from build123d import *

# Parameters (mm, degrees)
F0_R     = 2.1855866809
F1_DEPTH = 3.048


with BuildPart() as f1:
    # F0 (on Front) → F1 (new body)
    with BuildSketch(Plane.XZ):
        Polygon((-5.9369264533, -6.6248892115), (-8.0986570849, -26.090829358), (-8.0986570849, -29.0724959499), (-6.7978715524, -28.209612886), (-3.9593786933, -29.0724959499), (0, -28.209612886), (0, -5.0586252473), (4.1217724793, -0.9782924317), (1.2832815992, -8.4293344989), (5.1818756491, -2.3217138641), (1.8154965946, -11.4109388133), (5.7322757336, -6.8417807078), (2.702526981, -15.0221036917), (5.7322757336, -11.4109388133), (3.0573392287, -18.6332685701), (6.4980270698, -14.4673358305), (3.4121514764, -22.7992013097), (8.4402870655, -15.2195461217), (11.2180029973, -7.7197118662), (9.9174999541, 0), (5.0088027492, 10.0208651274), (8.024699986, 4.6986923553), (8.024699986, 10.0208651274), (9.9174999541, 2.5698228274), (9.9174999541, 8.0731014378), (12.9247023214, 1.6827941872), (12.9247023214, 7.682890673), (16.5401790291, 0), (16.5401790291, 5.5857207626), (18.9088093805, -2.7523501776), (18.9088093805, 2.0773874768), (21.6825364495, -3.8167845923), (21.6825364495, 0), (24.3970053162, -5.7682483457), (24.3970053162, 0), (21.6849464923, 5.7631270029), (17.9872654723, 10.3869775868), (13.3964173922, 12.7771075341), (7.8472970054, 15.6661421061), (14.1803448269, 14.6780370192), (12.2824395075, 15.6661421061), (20.1555828001, 13.5067671671), (16.00795798, 15.6661421061), (23.2676268034, 14.7984231008), (26.9920900816, 12.8593584523), (24.7008390725, 15.6661421061), (29.2833410908, 13.2803573629), (25.9918076559, 18.5046344995), (19.2012600601, 21.019651712), (14.9435270578, 21.019651712), (9.621351026, 21.019651712), (1.8154965946, 18.5046344995), (7.3503633432, 22.9420375162), (4.2991787195, 21.019651712), (7.6698875055, 25.0856313896), (2.8167848962, 22.9420375162), (9.621351026, 27.229225263), (4.6539907344, 27.229225263), (11.2102990657, 29.3158966176), (9.621351026, 29.9043957943), (12.7992471054, 31.9066156085), (9.621351026, 33.0836139619), (1.3918339066, 27.8986419471), (-2.087427536, 18.5046344995), (-3.3292702865, 24.9229501933), (-7.3300888762, 30.5999331176), (-14.4263189286, 35.2124832571), (-23.553526029, 35.2124832571), (-14.4263189286, 33.4919277449), (-19.5913599088, 33.4919277449), (-10.345986113, 30.0677157938), (-16.8121065944, 30.0677157938), (-8.8380374946, 25.5143014271), (-14.4263189286, 27.5840349495), (-7.3300888762, 22.9420375162), (-12.1995583177, 24.7455444187), (-7.3300888762, 21.019651712), (-4.5711095445, 15.6661421061), (-10.345986113, 21.019651712), (-17.1750385652, 23.54892998), (-25.8271690029, 22.7623730898), (-34.9033385476, 16.912889007), (-28.2102105994, 20.0625951825), (-31.419938263, 16.6290679), (-25.8271690029, 19.2609584022), (-27.8235962899, 17.1253293783), (-20.200404818, 20.7127123541), (-25.8271690029, 14.6936196567), (-16.2208060825, 19.2142594606), (-22.524728283, 14.6936196567), (-14.4263189286, 18.5046344995), (-18.0152932364, 14.6654174403), (-11.2330154516, 16.7931901649), (-15.135942027, 14.9565194733), (-7.3300888762, 15.6661421061), (-10.345986113, 14.2468968406), (-19.3936806172, 11.4084053785), (-27.2707313308, 5.2649948951), (-29.9890381223, -2.0744346548), (-29.9890381223, -10.8314546173), (-27.2713444978, -3.4936806187), (-27.2713444978, -7.5277050313), (-24.4833060582, 0), (-24.4833060582, -5.2881608668), (-22.524728283, 0), (-22.524728283, -3.4936806187), (-19.6370323027, 4.3030998167), (-17.7298966168, 0), (-15.4757376271, 6.086230278), (-15.4757376271, 1.2962748297), (-13.1431804335, 7.5941802934), (-12.4748563394, 6.086230278), (-16.0229708999, -3.4936806187), (-14.248913154, -15.3798665851), (-9.4963132998, -22.1003994255), (-12.4748563394, -15.3798665851), (-8.8154319776, -17.4274813299), (-12.4748563394, -9.1706654057), (-8.8154319776, -12.3146366909), (-11.3371305027, -6.6248892115), (-6.7978715524, -9.5822165707), (-9.4963132998, -3.4936806187), align=None)
        Polygon((-5.4590504354, -2.3217138641), (-5.9369264533, -6.6248892115), (-8.0986570849, 0), align=None, mode=Mode.SUBTRACT)
        Polygon((-5.2012195811, 0), (-5.4590504354, -2.3217138641), (-6.7978715524, 3.6025505979), align=None, mode=Mode.SUBTRACT)
        Polygon((4.1217724793, 2.9246343765), (0, -5.0586252473), (0, 0), align=None, mode=Mode.SUBTRACT)
        Polygon((-5.2116346857, 10.044903243), (-3.4663525091, 7.6787914149), (-4.0386512292, 7.6787914149), (-5.5632550193, 9.7079337566), (-6.0018647583, 9.318770627), (-6.0018647583, 7.6787914149), (-6.4880897508, 7.6787914149), (-6.4880897508, 11.8625239778), (-6.0018647583, 11.8625239778), (-6.0018647583, 9.7875977385), (-4.1045800417, 11.8625239778), (-3.5295342878, 11.8625239778), align=None, mode=Mode.SUBTRACT)
        Polygon((1.9929027185, 3.9890692569), (0, 0), (0, 1.9945346285), align=None, mode=Mode.SUBTRACT)
        with BuildLine():
            Line((0.8748766614, 7.6787914149), (0.482966498, 7.6787914149))
            Line((0.482966498, 7.6787914149), (-0.9363343277, 11.3872871207))
            Line((-0.9363343277, 11.3872871207), (-0.9592262765, 11.3872871207))
            add(Edge.make_bspline(
                [(-0.9592262765, 11.3872871207), (-0.9189364466, 10.9468460257), (-0.9189364466, 10.3397515435)],
                knots=[0, 0, 0, 1, 1, 1], degree=2))
            Line((-0.9189364466, 10.3397515435), (-0.9189364466, 7.6787914149))
            Line((-0.9189364466, 7.6787914149), (-1.368534321, 7.6787914149))
            Line((-1.368534321, 7.6787914149), (-1.368534321, 11.8625239778))
            Line((-1.368534321, 11.8625239778), (-0.6359919594, 11.8625239778))
            Line((-0.6359919594, 11.8625239778), (0.6889940372, 8.4113337766))
            Line((0.6889940372, 8.4113337766), (0.711885986, 8.4113337766))
            Line((0.711885986, 8.4113337766), (2.047860118, 11.8625239778))
            Line((2.047860118, 11.8625239778), (2.7749084119, 11.8625239778))
            Line((2.7749084119, 11.8625239778), (2.7749084119, 7.6787914149))
            Line((2.7749084119, 7.6787914149), (2.2886834194, 7.6787914149))
            Line((2.2886834194, 7.6787914149), (2.2886834194, 10.3745473057))
            add(Edge.make_bspline(
                [(2.2886834194, 10.3745473057), (2.2886834194, 10.8378803495), (2.3289732493, 11.381793053)],
                knots=[0, 0, 0, 1, 1, 1], degree=2))
            Line((2.3289732493, 11.381793053), (2.3060813005, 11.381793053))
            Line((2.3060813005, 11.381793053), (0.8748766614, 7.6787914149))
        make_face(mode=Mode.SUBTRACT)
        with Locations((-1.788830501, 14.6408742294)):
            Circle(F0_R, mode=Mode.SUBTRACT)
        Polygon((3.4916638397, -33.2978479564), (12.0071414858, -31.8786017597), (7.881906937, -29.8103850529), (6.8234760188, -30.6367613375), (6.1782777805, -29.8103850529), (5.1198468623, -30.6367613375), (3.8985372832, -29.0724959499), (1.8950107042, -30.6367613375), (0, -28.209612886), (-3.9593786933, -29.0724959499), (-6.7978715524, -28.209612886), (-8.0986570849, -29.0724959499), (-8.0986570849, -26.090829358), (-9.4963132998, -29.0724959499), (-11.3371305027, -28.209612886), (-12.4748563394, -30.6367613375), (-6.7978715524, -33.2978479564), align=None)
        Polygon((0, 0), (0, -5.0586252473), (4.1217724793, 2.9246343765), align=None)
        Polygon((-8.0986570849, 0), (-5.9369264533, -6.6248892115), (-5.4590504354, -2.3217138641), align=None)
    extrude(amount=F1_DEPTH)


solid = f1.part
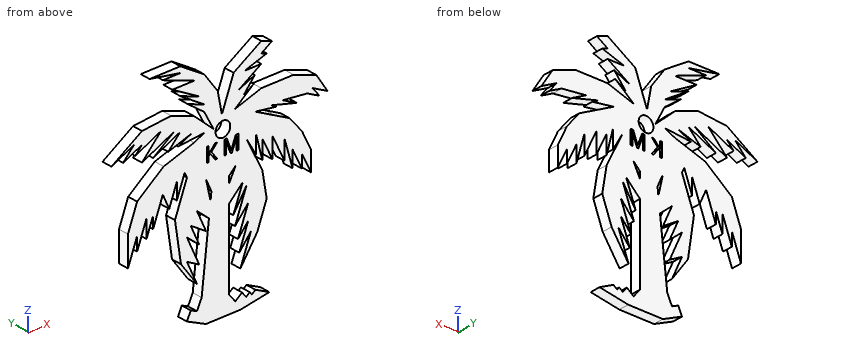
Work out the finished part from the listing and answer in its coordinate system (mm). Round coordinates to 2 decimals unless told otherwise and drop trailing zeros. Loops run counter-clockwise (first coordinate to the right, second up) from the corner with the lowest first, then second, coordinate; pieces in that order, holes last. Notation, with made-up numbers: (21.5, 41.25) - (38.5, 41.25) arc R20 cw to (38.5, 57.25) - close; hole circle Ø5 at (62, 3.25). An arc over 180 degrees is marked (long way). Use one line per item in the form item = value. Start each with the question number.
(1) Find section B-B on y = -0.9. Give the number of separate pieces and of enclosed holes in the cut face, and give its area (3 significant figures).
(2) Find section A-A on z = -16.5. Determine the outline of the cut face in (x, y).
(3) Flat-ended cylindrical pins translate along their axes: P1, Ø1.5, axis at y = -1, z = -1.5, coming from the +X side; P2, Ø1.5, axis at y = -2.5, z = -5, coming from the -X side; P3, Ø0.9, axis at y = -2, z = 7, coming from the +X side; P4, Ø2, axis at x = 7.5, z = -19.5, coming from the -Y side. Find the tip coordinate at first contact, or state that the pin passes through.
(4) Consider line 1 (X direction, y = -2, z = -11); line 2 (Z direction, x = 13, y = -2.3); line 3 (X direction, y = -0.2, z = -21). Determine where each line is inside the solid, lowest interval first.
Answer list:
q1.separate_pieces = 1
q1.enclosed_holes = 5
q1.area = 1,570 mm^2
q2.outline = (-13.46, -3.05) - (-11.98, -3.05) - (-11.98, 0) - (-13.46, 0) - close; (-10.47, -3.05) - (-9.23, -3.05) - (-9.23, 0) - (-10.47, 0) - close; (-7.03, -3.05) - (0, -3.05) - (0, 0) - (-7.03, 0) - close; (3.85, -3.05) - (4.82, -3.05) - (4.82, 0) - (3.85, 0) - close; (5.75, -3.05) - (7.59, -3.05) - (7.59, 0) - (5.75, 0) - close
q3.P1 = 24.4
q3.P2 = -29.99
q3.P3 = 21.06
q3.P4 = through
q4.line_1 = -14.9 to -11.66, -10.35 to -9.4, -6.42 to 0, 1.97 to 2.17, 4.19 to 10
q4.line_2 = 7.52 to 12.98, 14.86 to 15.29, 15.47 to 21.02
q4.line_3 = -10.27 to -9.98, -7.53 to 0, 4.08 to 4.61
